Read the model definition and answer for the solid it produces. Units are mm, in the model's axes. Face numbers are marked on the shaded views. Coordinates: 2 decimals unless noted, no trailing zeros. Loops run counter-clockwise (first coordinate to the right, second up) from the corner with the lowest first, then second, coordinate; pieces in that order, holes last. Notation, with made-up numbers: M 75.25,-1 L 128.25,-1 A28 cw 128.25,22 Z; hole C 57.25,20 d2. An arc over 180 degrees is marked long. Use one line per item in the form item = value. Start each with the question number.
1. For a pull along X with two mould halves and no side action, classify the marked faces 1, 2 and 3 as released by +X, released by -X, zero draft, split by the parting line, or undercut.
2. The part is cut by section A-A (y = 2.5). Give the vertices of the cut face in (x, z).
3. The part is cut by section B-B (x = 4.25). Give the vertices of the cut face in (y, z), plus the area to 3 significant figures.
4. Flat-ended cylindrical pins translate along their axes: pin 1 (4 mm diameter, centred on x = 3.5, y = 3.5, fed in from -Z); pin 2 (1.5 mm diameter, centred on y = 1, z = 2, fed in from +X). Find the tip coordinate at first contact, or state that the pin passes through.
5. Find the intervals of material crossed by probe 1 along Y at (x, z) = (3.5, 2.45); probe 2 along X at (y, z) = (3.25, 3.6); probe 3 along Y at (x, z) = (2.5, 0.8), in increasing order. Write a range as [from, to].
6. The part is cut by section D-D (y = 5.5). Give the vertices of the cut face in (x, z), plus the area to 3 significant figures.
7. The part is cut by section C-C (z = 0.7). Give the vertices of the cut face in (x, y), plus the area to 3 significant figures.
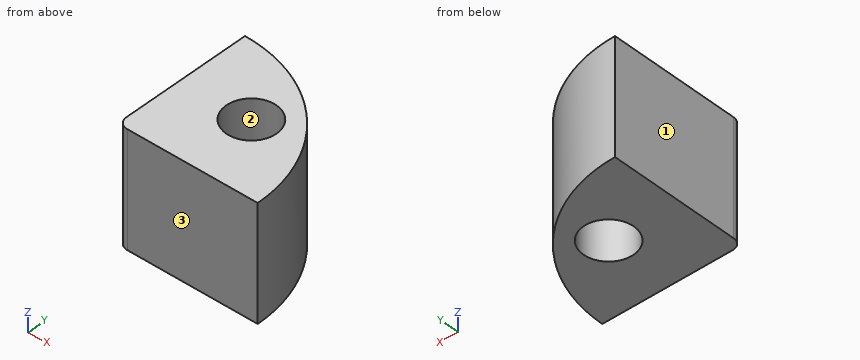
from build123d import *

# Parameters (mm, degrees)
P_IDAT_VYSUNUT_M1_DEPTH  = 5.7
SKICA2_R                 = 1.25
ODEBRAT_VYSUNUT_M1_DEPTH = 6.7
ZAOBLIT1_R               = 0.5


with BuildPart() as part:
    # Skica1 → Přidat vysunutím1 (new body)
    with BuildSketch(Plane.XY):
        with BuildLine():
            Line((0, 0), (7, 0))
            ThreePointArc((7, 0), (4.949747468, 4.949747468), (0, 7))
            Line((0, 7), (0, 0))
        make_face()
    extrude(amount=P_IDAT_VYSUNUT_M1_DEPTH)

    # Skica2 → Odebrat vysunutím1 (cut, through all)
    with BuildSketch(Plane.XY.offset(5.7)):
        with Locations((3.500178567, 3.500178567)):
            Circle(SKICA2_R)
    extrude(amount=-ODEBRAT_VYSUNUT_M1_DEPTH, mode=Mode.SUBTRACT)

    # Zaoblit1
    zaoblit1_edges = [part.edges().sort_by_distance(p)[0] for p in [
        (0, 0, 2.85),
    ]]
    fillet(zaoblit1_edges, radius=ZAOBLIT1_R)


solid = part.part
Computed values:
q1.face_1 = released by -X
q1.face_2 = undercut
q1.face_3 = zero draft
q2.outline = M 0,0 L 2.75,0 L 2.75,5.7 L 0,5.7 Z; M 4.25,0 L 6.54,0 L 6.54,5.7 L 4.25,5.7 Z
q3.outline = M 0,0 L 2.5,0 L 2.5,5.7 L 0,5.7 Z; M 4.5,0 L 5.56,0 L 5.56,5.7 L 4.5,5.7 Z
q3.area = 20.3 mm²
q4.pin_1 = 0
q4.pin_2 = 7
q5.probe_1 = [0, 2.25], [4.75, 6.06]
q5.probe_2 = [0, 2.28], [4.72, 6.2]
q5.probe_3 = [0, 2.75], [4.25, 6.54]
q6.outline = M 0,0 L 4.33,0 L 4.33,5.7 L 0,5.7 Z
q6.area = 24.7 mm²
q7.outline = M 0,0.5 A0.5 ccw 0.5,0 L 7,0 A7 ccw 0,7 Z; hole C 3.5,3.5 d2.5
q7.area = 33.5 mm²
